Design review of the part built by this model. Coordinates are the model's own, in mm. A direction names the side the tool comes from. Coordinates: 2 decimals unless noted, no trailing zeros. Write each loop counter-clockwise with the first axis right and the second up, starting at its lowest first coordinate (ties: lowest second). Pieces come first, ordered by that corner, then holes.
Q1. For L1, parallel to Z at x = 16, y = 0; L2, parallel to Y at x = 8.25, z = 0; L3, parallel to X at y = -8, z = -21.5, list the stretches that pass through material, from the lowest coordinate up.
Q2. Take a section at B-B, the plane z = 21. Write out the cut boundary in (x, y).
Q3. For faces 4 (the cylindrical face through (6.06, 28.33, 9.87)), 5 (the flat face through (10, 7, -7)), 6 (the cylindrical face through (6.056, 17.185, -2.055)), list the 3-axis set-ups (+Z, -Z, +X, -X, +Y, -Y) from which the entire face can be reached by the end or side of a thin tool; tool diameter is ignored.
Q4. The part is to be moulded in two halves that separate along Y. For faces 1 (the cylindrical face through (12.32, -1.85, -2.36)), 2 (the cylindrical face through (18.409, -0.867, -3.905)), 3 (the cylindrical face through (6.06, -28.33, -9.87)), say which applies: released by +Y, released by -Y, zero draft, split by the parting line, or undercut.
Q5. For pin 1 Ø1 at (y, z) = (-0.5, -25) entering from -X; pin 2 Ø8 at (y, z) = (1, -13) entering from +X; pin 3 Ø6 at (x, y) = (6, 1) entering from +Z, all flat-tipped, find the tip position at first contact; note any pin that passes through.
Q6. Take a section at C-C, the plane y = 17. Write out the cut boundary in (x, z).
Q7. Take a section at A-A, the plane x = 14.5. Write out the cut boundary in (y, z), plus the area to 3 significant figures.
from build123d import *

# Parameters (mm, degrees)
SKETCH3_W           = 10
SKETCH3_H           = 30
SKETCH4_R           = 3
CUT_EXTRUDE2_DEPTH  = 10
CUT_EXTRUDE3_START  = 2
SKETCH5_R           = 30
SKETCH5_R_2         = 4.5
CUT_EXTRUDE3_DEPTH  = 2
FILLET2_R           = 1.5
CUT_EXTRUDE6_START  = -8
CUT_EXTRUDE6_DEPTH  = 8
FILLET3_R           = 1.5
FILLET4_R           = 1
SKETCH11_R          = 32.5
SKETCH11_R_2        = 3
BOSS_EXTRUDE4_DEPTH = 2
SKETCH12_R          = 4
SKETCH12_R_2        = 3
BOSS_EXTRUDE5_DEPTH = 15


with BuildPart() as part:
    # Sketch3 → Revolve3 (revolve)
    with BuildSketch(Plane.XY):
        with Locations((5, 15)):
            Rectangle(SKETCH3_W, SKETCH3_H)
    revolve(axis=Axis((10, 0, 0), (-1, 0, 0)))

    # Sketch4 → Cut-Extrude2 (cut)
    with BuildSketch(Plane(origin=(0, 0, 0), x_dir=(0, 0, -1), z_dir=(1, 0, 0))):
        Circle(SKETCH4_R)
    extrude(amount=CUT_EXTRUDE2_DEPTH, mode=Mode.SUBTRACT)

    # Sketch5 → Cut-Extrude3 (cut)
    with BuildSketch(Plane(origin=(0, 0, 0), x_dir=(0, 0, -1), z_dir=(1, 0, 0)).offset(CUT_EXTRUDE3_START)):
        with Locations(Location((0, 0, 0), (0, 0, 90))):
            Circle(SKETCH5_R)
        Circle(SKETCH5_R_2, mode=Mode.SUBTRACT)
    extrude(amount=-CUT_EXTRUDE3_DEPTH, mode=Mode.SUBTRACT)

    # Fillet2
    fillet2_edges = [part.edges().sort_by_distance(p)[0] for p in [
        (0, 0, 4.5),
    ]]
    fillet(fillet2_edges, radius=FILLET2_R - 0.0001)  # a hair under: the kernel refuses the full size

    # Sketch6 → Cut-Extrude6 (cut)
    with BuildSketch(Plane.ZY.offset(-2).offset(CUT_EXTRUDE6_START)):
        with BuildLine():
            ThreePointArc((-3.911197191, -5.805388577), (-17.732937141, -1.783831627), (-29.187621061, 6.934174556))
            ThreePointArc((-29.187621061, 6.934174556), (-29.97689762, -1.177118976), (-28.554011024, -9.201546306))
            ThreePointArc((-28.554011024, -9.201546306), (-15.193906429, -10.611164811), (-2.377494131, -6.583883478))
            ThreePointArc((-2.377494131, -6.583883478), (-3.168347079, -6.241920921), (-3.911197191, -5.805388577))
        make_face()
        with BuildLine():
            ThreePointArc((-6.870663687, -1.339395574), (-13.800439543, 11.277720662), (-15.735562929, 25.54196663))
            ThreePointArc((-15.735562929, 25.54196663), (-22.029216396, 20.364518776), (-26.697210616, 13.684259035))
            ThreePointArc((-26.697210616, 13.684259035), (-18.246940863, 3.240487675), (-6.336650876, -2.974366432))
            ThreePointArc((-6.336650876, -2.974366432), (-6.654064316, -2.173344906), (-6.870663687, -1.339395574))
        make_face()
        with BuildLine():
            ThreePointArc((-25.54196663, -15.735562929), (-20.364518776, -22.029216396), (-13.684259035, -26.697210616))
            ThreePointArc((-13.684259035, -26.697210616), (-3.240487675, -18.246940863), (2.974366432, -6.336650876))
            ThreePointArc((2.974366432, -6.336650876), (2.173344906, -6.654064316), (1.339395574, -6.870663687))
            ThreePointArc((1.339395574, -6.870663687), (-11.277720662, -13.800439543), (-25.54196663, -15.735562929))
        make_face()
        with BuildLine():
            ThreePointArc((-6.934174556, -29.187621061), (1.177118976, -29.97689762), (9.201546306, -28.554011024))
            ThreePointArc((9.201546306, -28.554011024), (10.611164811, -15.193906429), (6.583883478, -2.377494131))
            ThreePointArc((6.583883478, -2.377494131), (6.241920921, -3.168347079), (5.805388577, -3.911197191))
            ThreePointArc((5.805388577, -3.911197191), (1.783831627, -17.732937141), (-6.934174556, -29.187621061))
        make_face()
        with BuildLine():
            ThreePointArc((15.735562929, -25.54196663), (22.029216396, -20.364518776), (26.697210616, -13.684259035))
            ThreePointArc((26.697210616, -13.684259035), (18.246940863, -3.240487675), (6.336650876, 2.974366432))
            ThreePointArc((6.336650876, 2.974366432), (6.654064316, 2.173344906), (6.870663687, 1.339395574))
            ThreePointArc((6.870663687, 1.339395574), (13.800439543, -11.277720662), (15.735562929, -25.54196663))
        make_face()
        with BuildLine():
            ThreePointArc((29.187621061, -6.934174556), (29.796213114, -3.49079992), (30, 0))
            ThreePointArc((30, 0), (29.636298105, 4.657234655), (28.554011024, 9.201546306))
            ThreePointArc((28.554011024, 9.201546306), (15.193906429, 10.611164811), (2.377494131, 6.583883478))
            ThreePointArc((2.377494131, 6.583883478), (3.168347079, 6.241920921), (3.911197191, 5.805388577))
            ThreePointArc((3.911197191, 5.805388577), (17.732937141, 1.783831627), (29.187621061, -6.934174556))
        make_face()
        with BuildLine():
            ThreePointArc((-1.339395574, 6.870663687), (11.277720662, 13.800439543), (25.54196663, 15.735562929))
            ThreePointArc((25.54196663, 15.735562929), (20.364518776, 22.029216396), (13.684259035, 26.697210616))
            ThreePointArc((13.684259035, 26.697210616), (3.240487675, 18.246940863), (-2.974366432, 6.336650876))
            ThreePointArc((-2.974366432, 6.336650876), (-2.173344906, 6.654064316), (-1.339395574, 6.870663687))
        make_face()
        with BuildLine():
            ThreePointArc((-5.805388577, 3.911197191), (-1.783831627, 17.732937141), (6.934174556, 29.187621061))
            ThreePointArc((6.934174556, 29.187621061), (-1.177118976, 29.97689762), (-9.201546306, 28.554011024))
            ThreePointArc((-9.201546306, 28.554011024), (-10.611164811, 15.193906429), (-6.583883478, 2.377494131))
            ThreePointArc((-6.583883478, 2.377494131), (-6.241920921, 3.168347079), (-5.805388577, 3.911197191))
        make_face()
    extrude(amount=CUT_EXTRUDE6_DEPTH, mode=Mode.SUBTRACT)

    # Fillet3
    fillet3_edges = [part.edges().sort_by_distance(p)[0] for p in [
        (6, 15.735562929, 25.54196663),
        (6, 29.187621061, 6.934174556),
        (6, 6.934174556, -29.187621061),
        (6, 25.54196663, -15.735562929),
        (6, -15.735562929, -25.54196663),
        (6, -29.187621061, -6.934174556),
        (6, -25.54196663, 15.735562929),
        (6, -6.934174556, 29.187621061),
    ]]
    fillet(fillet3_edges, radius=FILLET3_R)

    # Fillet4
    fillet4_edges = [part.edges().sort_by_distance(p)[0] for p in [
        (6, 26.697210616, 13.684259035),
        (6, 28.554011024, -9.201546306),
        (6, -9.201546306, -28.554011024),
        (6, 13.684259035, -26.697210616),
        (6, -26.697210616, -13.684259035),
        (6, -28.554011024, 9.201546306),
        (6, -13.684259035, 26.697210616),
        (6, 9.201546306, 28.554011024),
    ]]
    fillet(fillet4_edges, radius=FILLET4_R)

    # Sketch11 → Boss-Extrude4 (add)
    with BuildSketch(Plane(origin=(10, 0, 0), x_dir=(0, 0, -1), z_dir=(1, 0, 0))):
        with Locations(Location((0, 0, 0), (0, 0, 90))):
            Circle(SKETCH11_R)
        with Locations(Location((0, 0, 0), (0, 0, 90))):
            Circle(SKETCH11_R_2, mode=Mode.SUBTRACT)
    extrude(amount=BOSS_EXTRUDE4_DEPTH)

    # Sketch12 → Boss-Extrude5 (add)
    with BuildSketch(Plane(origin=(10, 0, 0), x_dir=(0, 0, -1), z_dir=(1, 0, 0))):
        with Locations(Location((0, 0, 0), (0, 0, 90))):
            Circle(SKETCH12_R)
        with Locations(Location((0, 0, 0), (0, 0, 90))):
            Circle(SKETCH12_R_2, mode=Mode.SUBTRACT)
    extrude(amount=BOSS_EXTRUDE5_DEPTH)


solid = part.part
Responses:
1. L1: z = -4 to -3, 3 to 4
1. L2: y = -20.9 to -13.5, -7.92 to -3, 3 to 7.92, 13.5 to 20.9
1. L3: x = 10 to 12
2. outline: (2, -5.77) - (10, -5.77) - (10, -24.8) - (12, -24.8) - (12, 24.8) - (10, 24.8) - (10, 15.7) - (2, 15.7) - (2, 10.68) - (10, 10.68) - (10, -0.06) - (2, -0.06) - close
3. face 4: +Z, -X, +Y
3. face 5: -X
3. face 6: -X, +Y
4. face 1: undercut
4. face 2: split by the parting line
4. face 3: released by -Y
5. pin 1: stops at x = 10
5. pin 2: stops at x = 12
5. pin 3: stops at z = 23.8
6. outline: (2, -15.22) - (10, -15.22) - (10, -27.7) - (12, -27.7) - (12, 27.7) - (10, 27.7) - (10, 2.27) - (2, 2.27) - (2, -2.14) - (10, -2.14) - (10, -10.74) - (2, -10.74) - close
7. outline: circle Ø8 at (0, 0); hole circle Ø6 at (0, 0)
7. area: 22.0 mm2
